The model under review builds one solid part; all positions refer to its coordinate system, in mm. Coordinates: 2 decimals unless noted, no trailing zeros. Order: outer loops, then holes, each group sorted by start corner. A loop starts at its lowest first (then second) coordinate and runs counter-clockwise, first axis right, second up. Notation, with made-up numbers: (15.25, 46.5) -> (40.25, 46.5) arc R16 cw to (40.25, 58.5) -> close; hole circle Ø3 at (-16.75, -1). An arc over 180 degrees is marked (long way). Use one line per item in the form item = value. Start each with the question number.
(1) Take a section at B-B (z = 88.8). State how many separate pieces and enclosed holes the cut face has, then the cut area to 3 significant figures.
(2) Wall thickness on line 1 along X through (y, z) = (7.75, 88.5); line 2 along Y through (x, z) = (-4.5, 87.7); line 3 along X through (y, z) = (-9.5, 87.1): over which ranges is each line inside the solid? List them lowest first.
(3) Take a section at C-C (x = -9.53). State the section outline as (y, z) points.
(4) Insertion check: pin 1 Ø8 at (x, y) = (70, 0) entering from -Z; pin 2 Ø1 at (x, z) = (32, 89) entering from +Y. Each pin has a flat end and moves straight along its axis. Give the tip position at first contact, or say it passes through.
(5) Take a section at A-A (x = 48). State the section outline as (y, z) points, then the cut area to 3 significant figures.
(6) Take a section at D-D (x = 27.5). State the section outline as (y, z) points.
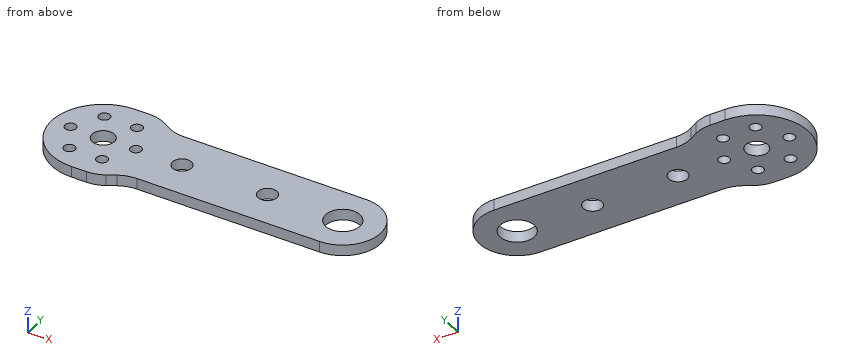
```python
from build123d import *

# Parameters (mm, degrees)
CROQUIS1_R                       = 5
CROQUIS1_R_2                     = 3.25
SALIENTE_EXTRUIR1_DEPTH          = 3.175
TALADRO_DE_MARGEN_PARA_41_D      = 3.2639
TALADRO_DE_MARGEN_PARA_41_DEPTH  = 10
TALADRO_DE_MARGEN_PARA_41_TIP    = 0.980574487
TALADRO_DE_MARGEN_PARA_M51_D     = 5.5
TALADRO_DE_MARGEN_PARA_M51_DEPTH = 6
TALADRO_DE_MARGEN_PARA_M51_TIP   = 1.652366702
REDONDEO1_R                      = 10


with BuildPart() as part:
    # Croquis1 → Saliente-Extruir1 (new body)
    with BuildSketch(Plane.XY.offset(86.203907482)):
        with BuildLine():
            Line((0, -15), (7, -15))
            Line((7, -15), (13.92820323, -11))
            Line((13.92820323, -11), (70, -11))
            ThreePointArc((70, -11), (81, 0), (70, 11))
            Line((70, 11), (13.92820323, 11))
            Line((13.92820323, 11), (7, 15))
            Line((7, 15), (0, 15))
            ThreePointArc((0, 15), (-15, 0), (0, -15))
        make_face()
        with Locations((70, 0)):
            Circle(CROQUIS1_R, mode=Mode.SUBTRACT)
        Circle(CROQUIS1_R_2, mode=Mode.SUBTRACT)
    extrude(amount=SALIENTE_EXTRUIR1_DEPTH)

    # Taladro de margen para #41
    with Locations(Plane.XY.offset(89.378907482)):
        with Locations((9.53, 0), (4.765, -8.253222098), (-4.765, -8.253222098), (-9.53, 0), (-4.765, 8.253222098), (4.765, 8.253222098)):
            Hole(TALADRO_DE_MARGEN_PARA_41_D / 2, depth=TALADRO_DE_MARGEN_PARA_41_DEPTH)
            with Locations((0, 0, -(TALADRO_DE_MARGEN_PARA_41_DEPTH + TALADRO_DE_MARGEN_PARA_41_TIP / 2))):  # 118° drill point
                Cone(0, TALADRO_DE_MARGEN_PARA_41_D / 2, TALADRO_DE_MARGEN_PARA_41_TIP, mode=Mode.SUBTRACT)

    # Taladro de margen para M51
    with Locations(Plane.XY.offset(89.378907482)):
        with Locations((23, 0), (48, 0)):
            Hole(TALADRO_DE_MARGEN_PARA_M51_D / 2, depth=TALADRO_DE_MARGEN_PARA_M51_DEPTH)
            with Locations((0, 0, -(TALADRO_DE_MARGEN_PARA_M51_DEPTH + TALADRO_DE_MARGEN_PARA_M51_TIP / 2))):  # 118° drill point
                Cone(0, TALADRO_DE_MARGEN_PARA_M51_D / 2, TALADRO_DE_MARGEN_PARA_M51_TIP, mode=Mode.SUBTRACT)

    # Redondeo1
    redondeo1_edges = [part.edges().sort_by_distance(p)[0] for p in [
        (7, 15, 87.791407482),
        (13.92820323, 11, 87.791407482),
        (13.92820323, -11, 87.791407482),
        (7, -15, 87.791407482),
    ]]
    fillet(redondeo1_edges, radius=REDONDEO1_R)


solid = part.part
```
Findings:
q1.separate_pieces = 1
q1.enclosed_holes = 10
q1.area = 1,960 mm²
q2.line_1 = -12.84 to -6.32, -3.21 to 3.21, 6.32 to 77.81
q2.line_2 = -14.31 to -9.86, -6.64 to 6.64, 9.86 to 14.31
q2.line_3 = -11.61 to -5.82, -3.71 to 3.71, 5.82 to 75.55
q3.outline = (-11.58, 86.2) -> (-1.63, 86.2) -> (-1.63, 89.38) -> (-11.58, 89.38) -> close; (1.63, 86.2) -> (11.58, 86.2) -> (11.58, 89.38) -> (1.63, 89.38) -> close
q4.pin_1 = through
q4.pin_2 = 11
q5.outline = (-11, 86.2) -> (-2.75, 86.2) -> (-2.75, 89.38) -> (-11, 89.38) -> close; (2.75, 86.2) -> (11, 86.2) -> (11, 89.38) -> (2.75, 89.38) -> close
q5.area = 52.4 mm²
q6.outline = (-11, 86.2) -> (11, 86.2) -> (11, 89.38) -> (-11, 89.38) -> close
